Autodesk Inventor part; units mm, degrees
ref_plane "YZ Plane" through (0, 0, 0) normal (1, 0, 0) x (0, 1, 0)
ref_plane "XZ Plane" through (0, 0, 0) normal (0, 1, 0) x (-1, 0, 0)
ref_plane "XY Plane" through (0, 0, 0) normal (0, 0, 1) x (1, 0, 0)
sketch "Sketch1" plane through (0, 0, 0) normal (0, 0, 1) x (1, 0, 0)
  line L0 (-101.6, 101.6) -> (-101.6, 0)
  arc A0 (-101.6, 0) -> (101.6, 0) centre (0, 0) ccw
  line L1 (101.6, 0) -> (101.6, 101.6)
  line L2 (-127, 101.6) -> (-127, 0)
  arc A1 (-127, 0) -> (127, 0) centre (0, 0) ccw
  line L3 (127, 0) -> (127, 101.6)
  line L4 (-127, 101.6) -> (-101.6, 101.6)
  line L5 (101.6, 101.6) -> (127, 101.6)
  dimension "d0" = 101.6
  dimension "d1" = 101.6
  dimension "d2" = 25.4
extrude "Extrusion1" add sketch "Sketch1" along normal mid plane 50.8
full round fillet "Fillet1" first side at (-110.0667, 33.8667, 25.4) centre faces at (110.0667, 101.6, -8.4667) second side at (-110.0667, 33.8667, -25.4)
full round fillet "Fillet2" first side at (-118.5333, 33.8667, 25.4) centre faces at (-118.5333, 101.6, 8.4667) second side at (-118.5333, 33.8667, -25.4)
hole "Hole1" at (127, 76.2, 0) direction (-1, 0, 0) diameter 25.4 end through all
properties part number "Forl"
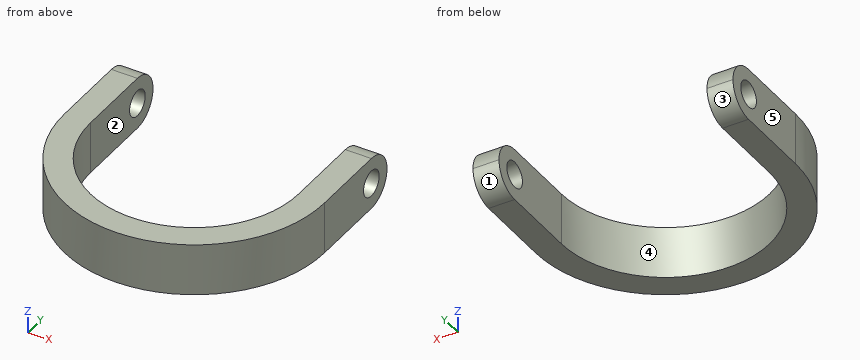
Geometry: final body of the model. Coordinates: model frame, mm. Face numbers are marked on the shaded views. A direction names the side the tool comes from. Round coordinates to 2 decimals unless told otherwise and drop trailing zeros. Order: outer loops, then holes, each group sorted by start corner. A loop starts at its lowest first (then second) coordinate and runs counter-clockwise, first axis right, second up. Notation, with made-up numbers: (66.5, 69.5) -> (99.5, 69.5) arc R30 ccw to (99.5, 92.5) -> close; hole circle Ø7 at (69, 21.5). An arc over 180 degrees is marked (long way). Use one line per item in the form item = value. Start each with the question number.
1. Cut plane D-D (x = 0). Return the cut outline in (y, z), then the cut area to 3 significant figures.
2. Pin query (flat end, axial travel): pin 1 Ø8 at (x, z) = (-86, 9) entering from +Y; pin 2 Ø20.5 at (y, z) = (76.2, 0) entering from -X; pin 3 Ø1.5 at (x, z) = (-21, -1.5) entering from +Y; pin 4 Ø4 at (x, z) = (-20, -18.5) entering from -Y. Return the tip coordinate at first contact, or that it passes through.
3. Draft query along X for the marked faces 3, 4 and 5. Return one class per face: pulls with the +X half, pulls with the -X half, needs draft (parallel to the pull), parting line crosses it, or undercut.
4. Cut plane C-C (z = -21). Return the cut outline in (x, y), then the cut area to 3 significant figures.
5. Reachability of the marked faces 1 and 2 from +Z, -Z, +X, -X, +Y, -Y: full face, straight path, thin tool, end or side. Return the list, or none.
6. Cut plane A-A (z = -8.5). Return the cut outline in (x, y), then the cut area to 3 significant figures.
7. Line query: probe 1 along Z at (x, y) = (111, 76); probe 2 along X at (y, z) = (63, -7.5); probe 3 along X at (y, z) = (-12.5, 14.5). Output: solid intervals per line, ascending.
Solution:
q1.outline = (-127, -25.4) -> (-101.6, -25.4) -> (-101.6, 25.4) -> (-127, 25.4) -> close
q1.area = 1,290 mm^2
q2.pin_1 = -47.14
q2.pin_2 = through
q2.pin_3 = -99.24
q2.pin_4 = -125.72
q3.face_3 = needs draft
q3.face_4 = undercut
q3.face_5 = pulls with the -X half
q4.outline = (-127, 0) arc R127 ccw to (127, 0) -> (127, 90.49) -> (101.6, 90.49) -> (101.6, 0) arc R101.6 cw to (-101.6, 0) -> (-101.6, 90.49) -> (-127, 90.49) -> close
q4.area = 13,700 mm^2
q5.face_1 = -Z, +X, -X, +Y
q5.face_2 = +Z, -Z, +Y
q6.outline = (-127, 0) arc R127 ccw to (127, 0) -> (127, 66.76) -> (101.6, 66.76) -> (101.6, 0) arc R101.6 cw to (-101.6, 0) -> (-101.6, 66.76) -> (-127, 66.76) -> close; (-127, 85.64) -> (-101.6, 85.64) -> (-101.6, 100.14) -> (-127, 100.14) -> close; (101.6, 85.64) -> (127, 85.64) -> (127, 100.14) -> (101.6, 100.14) -> close
q6.area = 13,200 mm^2
q7.probe_1 = -25.4 to -12.7, 12.7 to 25.4
q7.probe_2 = -127 to -101.6, 101.6 to 127
q7.probe_3 = -126.38 to -100.83, 100.83 to 126.38
